Could you check a few things on this model? Use its own coordinates, in mm. A direction names the side the tool comes from. Give positions to 0.01 mm unless a question says otherwise; leave off trailing zeros. Order: outer loops, then holes, each group sorted by start corner. A loop starts at its lowest first (then second) coordinate and runs counter-clockwise, first axis right, second up.
from build123d import *

# Parameters (mm, degrees)
SKETCH1_R           = 10
BOSS_EXTRUDE1_DEPTH = 3
SKETCH2_R           = 3
BOSS_EXTRUDE2_DEPTH = 5.5
CUT_EXTRUDE1_DEPTH  = 4.5
CUT_EXTRUDE2_DEPTH  = 2
FILLET3_R           = 0.6
CHAMFER1_SIZE       = 1
FILLET4_START       = -0.303359817
FILLET4_2_DEPTH     = 0.303359817


with BuildPart() as part:
    # Sketch1 → Boss-Extrude1 (new body)
    with BuildSketch(Plane(origin=(0, 0, 0), x_dir=(1, 0, 0), z_dir=(0, 1, 0))):
        with Locations(Location((0, 0, 0), (0, 0, 270))):
            Circle(SKETCH1_R)
    extrude(amount=BOSS_EXTRUDE1_DEPTH)

    # Sketch2 → Boss-Extrude2 (add)
    with BuildSketch(Plane.XZ):
        with Locations(Location((0, 0, 0), (0, 0, 90))):
            Circle(SKETCH2_R)
    extrude(amount=BOSS_EXTRUDE2_DEPTH)

    # Sketch3 → Cut-Extrude1 (cut)
    with BuildSketch(Plane.XZ.offset(5.5)):
        Polygon((0.55, 0.55), (5.536201487, 0.55), (5.536201487, -0.65), (0.55, -0.65), (0.55, -5.164287365), (-0.65, -5.164287365), (-0.65, -0.65), (-5.536201487, -0.65), (-5.536201487, 0.55), (-0.65, 0.55), (-0.65, 5.164287365), (0.55, 5.164287365), align=None)
    extrude(amount=-CUT_EXTRUDE1_DEPTH, mode=Mode.SUBTRACT)

    # Sketch4 → Cut-Extrude2 (cut)
    with BuildSketch(Plane.XZ):
        with BuildLine():
            Line((-0.834967988, 6.279069136), (-0.347460476, 5.81308022))
            add(Edge.make_bspline(
                [(-0.347460476, 5.81308022), (-0.306106117, 5.855840696), (-0.225328099, 5.939365303), (-0.095164312, 6.049944522), (0.040201287, 6.142097338), (0.178135431, 6.219707854), (0.321119155, 6.27842574), (0.467499177, 6.321214453), (0.618210178, 6.347301114), (0.720205587, 6.350285889), (0.771506538, 6.351787151)],
                knots=[0, 0, 0, 0, 1.115251505, 2.178435587, 3.19620269, 4.182487026, 5.141301733, 6.088180966, 7.038406374, 8, 8, 8, 8], degree=3))
            add(Edge.make_bspline(
                [(0.771506538, 6.351787151), (0.814349066, 6.350601102), (0.898894076, 6.348260564), (1.023028305, 6.331102112), (1.14176911, 6.301923419), (1.255522961, 6.261709774), (1.363955131, 6.209675452), (1.467292962, 6.145860726), (1.565281679, 6.070841933), (1.656626907, 5.985007225), (1.740186311, 5.891226356), (1.814016366, 5.791162393), (1.87586088, 5.685044577), (1.926615666, 5.57394759), (1.966151683, 5.45735722), (1.994385366, 5.335351962), (2.010714974, 5.207786517), (2.013152277, 5.121068477), (2.014390986, 5.076995818)],
                knots=[0, 0, 0, 0, 1.035432265, 2.043311493, 3.022114605, 3.98653278, 4.95457646, 5.923598177, 6.917315552, 7.932509744, 8.948865224, 9.949768934, 10.933144597, 11.912367597, 12.897413939, 13.903909035, 14.934704909, 16, 16, 16, 16], degree=3))
            add(Edge.make_bspline(
                [(2.014390986, 5.076995818), (2.014034004, 5.046062543), (2.013330386, 4.985092421), (2.005628036, 4.89490069), (1.993225435, 4.807393388), (1.9752758, 4.722703065), (1.952829605, 4.64075633), (1.926495106, 4.56084623), (1.893458866, 4.484076944), (1.85678814, 4.409556847), (1.814140509, 4.339319312), (1.768158495, 4.272341994), (1.718298508, 4.208953207), (1.664237603, 4.149412088), (1.605214938, 4.094649132), (1.542756032, 4.04301755), (1.47580729, 3.995809856), (1.405759405, 3.95184132), (1.332007254, 3.91364548), (1.256551903, 3.879047428), (1.178249297, 3.850948665), (1.098052816, 3.828298499), (1.016249056, 3.809037916), (0.932037899, 3.797178583), (0.84614935, 3.788197649), (0.788103108, 3.787643128), (0.758892188, 3.787364074)],
                knots=[0, 0, 0, 0, 1.103660481, 2.175337485, 3.227646561, 4.255952547, 5.262355991, 6.258840057, 7.255597736, 8.242457506, 9.22035537, 10.185017736, 11.140346927, 12.096287581, 13.051739095, 14.01125915, 14.986044842, 15.97314143, 16.960198552, 17.947847494, 18.933482797, 19.925264591, 20.920966487, 21.929612487, 22.958107872, 24, 24, 24, 24], degree=3))
            add(Edge.make_bspline(
                [(0.758892188, 3.787364074), (0.709345449, 3.788797229), (0.611998989, 3.791613005), (0.469129063, 3.813631976), (0.332988257, 3.849851938), (0.224212405, 3.892625607), (0.138989397, 3.934865162), (0.074110382, 3.973934669), (0.007020423, 4.017638203), (-0.061166173, 4.067625182), (-0.131216368, 4.123295742), (-0.201893616, 4.185869172), (-0.275007267, 4.253285019), (-0.322903296, 4.301401034), (-0.347460476, 4.326071005)],
                knots=[0, 0, 0, 0, 1.404581149, 2.759636711, 4.088442092, 5.392261763, 6.066678138, 6.783632037, 7.538459478, 8.336747902, 9.180226004, 10.074962426, 11.012997595, 12, 12, 12, 12], degree=3))
            Line((-0.347460476, 4.326071005), (-0.820127577, 3.829659247))
            add(Edge.make_bspline(
                [(-0.820127577, 3.829659247), (-0.786901624, 3.797580632), (-0.722051669, 3.734970037), (-0.624227313, 3.646068834), (-0.526526072, 3.56618122), (-0.431308206, 3.492407626), (-0.337013946, 3.426897254), (-0.243653292, 3.36958468), (-0.152283128, 3.319020385), (-0.061006122, 3.276057111), (0.030745698, 3.239576829), (0.125147538, 3.208169701), (0.222487994, 3.181600401), (0.323361577, 3.160162465), (0.426827399, 3.142972134), (0.533853763, 3.13136876), (0.64376207, 3.123568198), (0.718314577, 3.122867253), (0.755924106, 3.122513647)],
                knots=[0, 0, 0, 0, 1.244526981, 2.429050516, 3.560637417, 4.644440555, 5.67424972, 6.652764056, 7.595344123, 8.486817594, 9.369275933, 10.254498637, 11.166417451, 12.086725134, 13.032340136, 13.991389299, 14.986715468, 16, 16, 16, 16], degree=3))
            add(Edge.make_bspline(
                [(0.755924106, 3.122513647), (0.825008152, 3.124274737), (0.960186427, 3.127720701), (1.158286664, 3.15325296), (1.346476572, 3.196057342), (1.525213981, 3.256594544), (1.694442057, 3.333927983), (1.854117507, 3.428735148), (2.003982968, 3.540764151), (2.142827823, 3.668701904), (2.268419602, 3.809998412), (2.379428191, 3.961712098), (2.4712545, 4.124588579), (2.547499862, 4.29622165), (2.607122733, 4.477394539), (2.649087127, 4.668303219), (2.674966262, 4.868763357), (2.677797476, 5.005682252), (2.679241414, 5.075511777)],
                knots=[0, 0, 0, 0, 1.078019885, 2.10938526, 3.111377082, 4.085535484, 5.04941344, 6.010039228, 6.978205633, 7.964457913, 8.951525778, 9.924444315, 10.892603023, 11.863865945, 12.85144698, 13.863884204, 14.910567087, 16, 16, 16, 16], degree=3))
            add(Edge.make_bspline(
                [(2.679241414, 5.075511777), (2.678631276, 5.121053998), (2.677422131, 5.211307547), (2.664713911, 5.344258338), (2.646997912, 5.473861578), (2.618893092, 5.598771556), (2.585015503, 5.720671039), (2.54288427, 5.838235123), (2.492566683, 5.951801699), (2.435684595, 6.061560883), (2.371334459, 6.166793637), (2.299448292, 6.266595843), (2.221876725, 6.361737958), (2.136755839, 6.450957744), (2.045322553, 6.535038569), (1.947164056, 6.613524781), (1.842870722, 6.687541963), (1.732160268, 6.755181391), (1.617183502, 6.816364849), (1.499390586, 6.870331271), (1.379070921, 6.915434773), (1.256733231, 6.952846464), (1.13186064, 6.980771646), (1.005344457, 7.001910108), (0.876108181, 7.013726643), (0.789337218, 7.015661085), (0.745535818, 7.016637579)],
                knots=[0, 0, 0, 0, 1.071919942, 2.124283339, 3.142214191, 4.149696895, 5.136002878, 6.119640489, 7.086990633, 8.058538607, 9.028339693, 9.988281803, 10.952401235, 11.916291999, 12.888973767, 13.874849856, 14.873389453, 15.898127285, 16.927174885, 17.938320013, 18.946391617, 19.950418109, 20.947802303, 21.956882652, 22.968648068, 24, 24, 24, 24], degree=3))
            add(Edge.make_bspline(
                [(0.745535818, 7.016637579), (0.708168733, 7.016077828), (0.633823076, 7.014964147), (0.523109917, 7.005680404), (0.41328219, 6.99110038), (0.304733111, 6.969102228), (0.196686228, 6.942987643), (0.090561397, 6.908794195), (-0.015315558, 6.870679153), (-0.119284115, 6.825120403), (-0.221489399, 6.775388913), (-0.319537089, 6.718966731), (-0.415073398, 6.659326016), (-0.505981298, 6.592936968), (-0.59396369, 6.522207642), (-0.678560506, 6.446808046), (-0.75902936, 6.365481048), (-0.809527145, 6.308018722), (-0.834967988, 6.279069136)],
                knots=[0, 0, 0, 0, 0.996412454, 1.982464992, 2.961075852, 3.949442424, 4.934965278, 5.923860011, 6.921385422, 7.934793307, 8.949617135, 9.951082467, 10.950285876, 11.951772932, 12.951063433, 13.960125323, 14.972308753, 16, 16, 16, 16], degree=3))
        make_face()
        Polygon((-1.452329099, 7.016637579), (-2.117179526, 7.016637579), (-2.117179526, 5.924383305), (-2.544583373, 5.924383305), (-2.544583373, 5.35451151), (-2.117179526, 5.35451151), (-2.117179526, 3.217492279), (-1.452329099, 3.217492279), (-1.452329099, 5.35451151), (-1.119903885, 5.35451151), (-1.119903885, 5.924383305), (-1.452329099, 5.924383305), align=None)
    extrude(amount=-CUT_EXTRUDE2_DEPTH, mode=Mode.SUBTRACT)

    # Fillet3
    fillet3_edges = [part.edges().sort_by_distance(p)[0] for p in [
        (1.74957621, -5.5, 0.55),
        (-0.65, -5.5, 1.739368465),
        (-1.789368465, -5.5, -0.65),
        (0.55, -5.5, -1.79957621),
        (0.55, -5.5, 1.74957621),
        (-1.79957621, -5.5, 0.55),
        (-0.65, -5.5, -1.789368465),
        (1.739368465, -5.5, -0.65),
    ]]
    fillet(fillet3_edges, radius=FILLET3_R)

    # Chamfer1
    chamfer1_edges = [part.edges().sort_by_distance(p)[0] for p in [
        (0, 3, -10),
    ]]
    chamfer(chamfer1_edges, length=CHAMFER1_SIZE)

    # Fillet4: read off the stored shape, not the designer's step
    # Fillet4 outline → Fillet4 (revolve)
    with BuildSketch(Plane.XY):
        with BuildLine():
            ThreePointArc((3, -0.8), (3.234314575, -0.234314575), (3.8, 0))
            Line((3.8, 0), (3, 0))
            Line((3, 0), (3, -0.8))
        make_face()
    revolve(axis=Axis((0, 0, 0), (0, 1, 0)))

    # Fillet4 2 outline → Fillet4 2 (cut)
    with BuildSketch(Plane(origin=(0, 0, 0), x_dir=(1, 0, 0), z_dir=(0, 1, 0)).offset(FILLET4_START)):
        with BuildLine():
            Line((-1.452329099, -3.511515369), (-1.452329099, -3.217492279))
            Line((-1.452329099, -3.217492279), (-2.021816864, -3.217492279))
            ThreePointArc((-2.021816864, -3.217492279), (-1.743282805, -3.376531514), (-1.452329099, -3.511515369))
        make_face()
        with BuildLine():
            add(Edge.make_bspline(
                [(-0.717504439, -3.731646738), (-0.686203446, -3.702392774), (-0.623361366, -3.645360773), (-0.526526072, -3.56618122), (-0.431308206, -3.492407626), (-0.337013946, -3.426897254), (-0.243653292, -3.36958468), (-0.152283128, -3.319020385), (-0.061006122, -3.276057111), (0.030745698, -3.239576829), (0.125147538, -3.208169701), (0.222487994, -3.181600401), (0.323361577, -3.160162465), (0.426827399, -3.142972134), (0.533853763, -3.13136876), (0.64376207, -3.123568198), (0.718314577, -3.122867253), (0.755924106, -3.122513647)],
                knots=[0.079666321, 0.079666321, 0.079666321, 0.079666321, 0.151815657, 0.222539839, 0.290277535, 0.354640607, 0.415797753, 0.474709008, 0.5304261, 0.585579746, 0.640906165, 0.697901091, 0.755420321, 0.814521258, 0.874461831, 0.936669717, 1, 1, 1, 1], degree=3))
            ThreePointArc((-0.717504439, -3.731646738), (0.549009685, -3.760131429), (1.754506577, -3.370713081))
            add(Edge.make_bspline(
                [(0.755924106, -3.122513647), (0.825008152, -3.124274737), (0.960186427, -3.127720701), (1.158286664, -3.15325296), (1.346476572, -3.196057342), (1.525213981, -3.256594544), (1.659634947, -3.318021913), (1.73426641, -3.359048476), (1.754506577, -3.370713081)],
                knots=[0, 0, 0, 0, 0.067376243, 0.131836579, 0.194461068, 0.255345968, 0.31558834, 0.33836485, 0.33836485, 0.33836485, 0.33836485], degree=3))
        make_face()
    extrude(amount=FILLET4_2_DEPTH, mode=Mode.SUBTRACT)


solid = part.part
Item 1: For faces 4 (the flat face through (0.55, -3, 2)), 5 (the flat face through (2, 2, 6)), 6 (the flat face through (0, 3, 0)), 7 (the flat face through (2, -3, 0.55)), which set-ups out of +Z, -Z, +X, -X, +Y, -Y let a thin tool reach every point of the face, with its end or its side?
Findings:
face 4: +Z, -Z, -Y
face 5: -Y
face 6: +Z, -Z, +X, -X, +Y
face 7: +X, -X, -Y
Item 2: We'd pull the mould along Z, two halves only. Please class faces 1 (the flat face through (-2.117, 1, 4)), 2 (the flat face through (-2, -5.5, -2)), 3 (the cylindrical face through (-9.76, 0.99, -2.17)): +Z half, -Z half, draft (parallel to the pull), parting line (faces both ways), or undercut.
Findings:
face 1: undercut
face 2: draft
face 3: parting line
Item 3: Imagine slicing it at A-A on y = -2. List the corners of the cut face in (x, z) for me.
Findings:
outline: (-2.95, 0.55) - (-0.65, 0.55) - (-0.65, 2.93) arc R3 ccw to start; (-2.93, -0.65) arc R3 ccw to (-0.65, -2.93) - (-0.65, -0.65) - close; (0.55, -2.95) arc R3 ccw to (2.93, -0.65) - (0.55, -0.65) - close; (0.55, 0.55) - (2.95, 0.55) arc R3 ccw to (0.55, 2.95) - close
Item 4: For pin 1 (0.6 mm diameter, centred on y = 1, z = 4, fed in from -X); pin 2 (2 mm diameter, centred on x = 2.5, y = -3.5, fed in from -Z); pin 3 (0.5 mm diameter, centred on y = 1, z = 5.5, fed in from +X); pin 4 (5 mm diameter, centred on y = 0.5, z = 0.5, fed in from -X), each with a flat end and sliding along its axis, tell me the tip position at first contact or that it passes through.
Findings:
pin 1: stops at x = -9.29
pin 2: stops at z = -2.6
pin 3: stops at x = 8.51
pin 4: stops at x = -10
Item 5: Please list where these lines run through material, in increasing order: line 1 along Y through (x, z) = (0.5, 5.25); line 2 along Z through (x, y) = (0.5, 0.5); line 3 along Y through (x, z) = (0.5, -0.75).
Findings:
line 1: y = 0 to 3
line 2: z = -9.99 to 3.14, 3.81 to 6.33, 7 to 9.99
line 3: y = -1 to 3
Item 6: Imagine slicing it at B-B on z = 0. List the corners of the cut face in (x, y) for me.
Findings:
outline: (-10, 0) - (-3.8, 0) arc R0.8 cw to (-3, -0.8) - (-3, -1) - (3, -1) - (3, -0.8) arc R0.8 cw to (3.8, 0) - (10, 0) - (10, 2) - (9, 3) - (-9, 3) - (-10, 2) - close
Item 7: Imagine slicing it at C-C on y = 0.75. Give the number of separate pieces and of enclosed holes in the cut face, then the cut area to 3 significant figures.
Findings:
separate pieces: 1
enclosed holes: 2
area: 306 mm2
